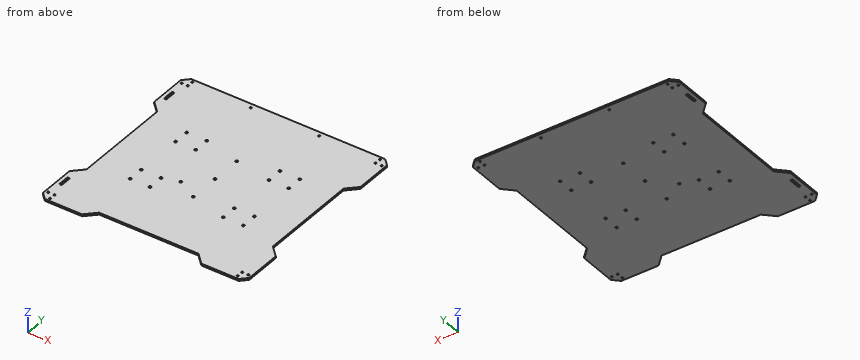
```python
from build123d import *

# Parameters (mm, degrees)
SKETCH1_R           = 2
SKETCH1_R_2         = 1.5
BOSS_EXTRUDE1_DEPTH = 3.175
CUT_EXTRUDE1_DEPTH  = 4.175
CHAMFER1_SIZE       = 10


with BuildPart() as part:
    # Sketch1 → Boss-Extrude1 (new body)
    with BuildSketch(Plane.XY):
        Polygon((166, 166), (166, 96), (150, 80), (150, -80), (166, -96), (166, -166), (96, -166), (80, -150), (-80, -150), (-96, -166), (-166, -166), (-166, -96), (-150, -80), (-150, 80), (-166, 96), (-166, 166), align=None)
        with Locations((-91, 64)):
            Circle(SKETCH1_R, mode=Mode.SUBTRACT)
        with Locations((-91, 39)):
            Circle(SKETCH1_R, mode=Mode.SUBTRACT)
        with Locations((-59, 39)):
            Circle(SKETCH1_R, mode=Mode.SUBTRACT)
        with Locations((-59, 64)):
            Circle(SKETCH1_R, mode=Mode.SUBTRACT)
        with Locations((59, 39)):
            Circle(SKETCH1_R, mode=Mode.SUBTRACT)
        with Locations((59, 64)):
            Circle(SKETCH1_R, mode=Mode.SUBTRACT)
        with Locations((91, 39)):
            Circle(SKETCH1_R, mode=Mode.SUBTRACT)
        with Locations((91, 64)):
            Circle(SKETCH1_R, mode=Mode.SUBTRACT)
        with Locations((59, -64)):
            Circle(SKETCH1_R, mode=Mode.SUBTRACT)
        with Locations((59, -39)):
            Circle(SKETCH1_R, mode=Mode.SUBTRACT)
        with Locations((91, -39)):
            Circle(SKETCH1_R, mode=Mode.SUBTRACT)
        with Locations((91, -64)):
            Circle(SKETCH1_R, mode=Mode.SUBTRACT)
        with Locations((-91, -64)):
            Circle(SKETCH1_R, mode=Mode.SUBTRACT)
        with Locations((-59, -64)):
            Circle(SKETCH1_R, mode=Mode.SUBTRACT)
        with Locations((-59, -39)):
            Circle(SKETCH1_R, mode=Mode.SUBTRACT)
        with Locations((-91, -39)):
            Circle(SKETCH1_R, mode=Mode.SUBTRACT)
        with Locations((-33, -31)):
            Circle(SKETCH1_R, mode=Mode.SUBTRACT)
        Circle(SKETCH1_R, mode=Mode.SUBTRACT)
        with Locations((0, 49)):
            Circle(SKETCH1_R, mode=Mode.SUBTRACT)
        with Locations((0, -49)):
            Circle(SKETCH1_R, mode=Mode.SUBTRACT)
        with Locations((-151, 161)):
            Circle(SKETCH1_R_2, mode=Mode.SUBTRACT)
        with Locations((-161, 151)):
            Circle(SKETCH1_R_2, mode=Mode.SUBTRACT)
        with Locations((151, 161)):
            Circle(SKETCH1_R_2, mode=Mode.SUBTRACT)
        with Locations((161, 151)):
            Circle(SKETCH1_R_2, mode=Mode.SUBTRACT)
        with Locations((161, -151)):
            Circle(SKETCH1_R_2, mode=Mode.SUBTRACT)
        with Locations((151, -161)):
            Circle(SKETCH1_R_2, mode=Mode.SUBTRACT)
        with Locations((-151, -161)):
            Circle(SKETCH1_R_2, mode=Mode.SUBTRACT)
        with Locations((-161, -151)):
            Circle(SKETCH1_R_2, mode=Mode.SUBTRACT)
        with Locations((-151, 151)):
            Circle(SKETCH1_R_2, mode=Mode.SUBTRACT)
        with Locations((151, 151)):
            Circle(SKETCH1_R_2, mode=Mode.SUBTRACT)
        with Locations((151, -151)):
            Circle(SKETCH1_R_2, mode=Mode.SUBTRACT)
        with Locations((-151, -151)):
            Circle(SKETCH1_R_2, mode=Mode.SUBTRACT)
        with Locations((-55, 158.5)):
            Circle(SKETCH1_R_2, mode=Mode.SUBTRACT)
        with Locations((55, 158.5)):
            Circle(SKETCH1_R_2, mode=Mode.SUBTRACT)
    extrude(amount=BOSS_EXTRUDE1_DEPTH)

    # Sketch2 → Cut-Extrude1 (cut, through all)
    with BuildSketch(Plane.XY.offset(3.175)):
        with BuildLine():
            Line((-160, 126), (-160, 111))
            ThreePointArc((-160, 111), (-158, 109), (-156, 111))
            Line((-156, 111), (-156, 126))
            ThreePointArc((-156, 126), (-158, 128), (-160, 126))
        make_face()
        with BuildLine():
            Line((-156, -111), (-156, -126))
            ThreePointArc((-156, -126), (-158, -128), (-160, -126))
            Line((-160, -126), (-160, -111))
            ThreePointArc((-160, -111), (-158, -109), (-156, -111))
        make_face()
    extrude(amount=-CUT_EXTRUDE1_DEPTH, mode=Mode.SUBTRACT)

    # Chamfer1
    chamfer1_edges = [part.edges().sort_by_distance(p)[0] for p in [
        (166, -166, 1.5875),
        (-166, -166, 1.5875),
        (-166, 166, 1.5875),
        (166, 166, 1.5875),
    ]]
    chamfer(chamfer1_edges, length=CHAMFER1_SIZE)


solid = part.part
```
Model file for the job. Use its own axes, mm. Coordinates: 2 decimals unless noted, no trailing zeros. Write each loop counter-clockwise with the first axis right and the second up, starting at its lowest first coordinate (ties: lowest second). Pieces come first, ordered by that corner, then holes. Notation, with made-up numbers: (60.5, -14) - (112.5, -14) arc R24 cw to (112.5, 9) - close; hole circle Ø1 at (-33.5, -1.5). An arc over 180 degrees is marked (long way). One line per question, with ' | ' between items. Start each with the question number.
Q1. Cut at A-A, the plane z = 1.8. Give the number of separate pieces and of enclosed holes in the cut face, then the cut area to 3 significant figures.
Q2. Cut at B-B, the plane x = 74. List the corners of the cut face in (y, z) (3 decimals).
Q3. Drill centre lines: line 1 (X direction, y = 151, z = 2.35); line 2 (Y direction, x = -33, z = 1.8); line 3 (Y direction, x = -151, z = 2.4). Where is each one in solid material? Low to high. Write a range as [from, to].
Q4. Pin check, flat tips, straight feed: pin 1 (3.5 mm diameter, centred on x = -91, y = -39, fed in from +Z); pin 2 (1 mm diameter, centred on y = 72.5, z = 1.5, fed in from +X). Stop position of each tip, or through.
Q5. Cut at C-C, the plane y = -8. List the corners of the cut face in (x, z) (3 decimals), then the cut area to 4 significant figures.
Answer below:
1) separate pieces: 1 | enclosed holes: 36 | area: 101,000 mm^2
2) outline: (-150, 0) - (166, 0) - (166, 3.175) - (-150, 3.175) - close
3) line 1: [-166, -162.5], [-159.5, -152.5], [-149.5, 149.5], [152.5, 159.5], [162.5, 166] | line 2: [-150, -33], [-29, 166] | line 3: [-166, -162.5], [-159.5, -152.5], [-149.5, -81], [81, 149.5], [152.5, 159.5], [162.5, 166]
4) pin 1: through | pin 2: x = 150
5) outline: (-150, 0) - (150, 0) - (150, 3.175) - (-150, 3.175) - close | area: 952.5 mm^2
